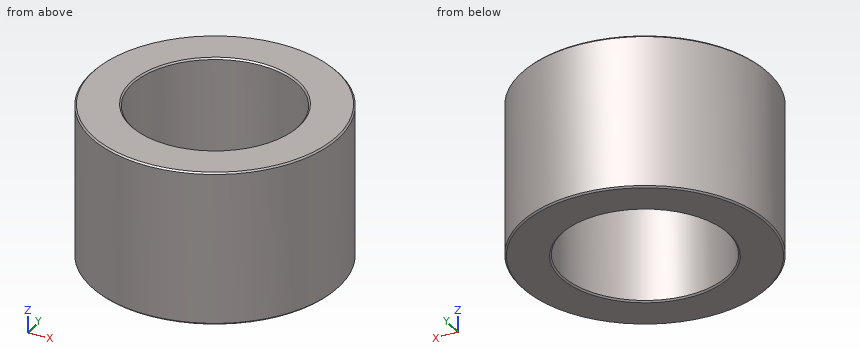
```python
from build123d import *

# Parameters (mm, degrees)
F0_R     = 40.239299
F1_DEPTH = 50
F2_R     = 26.870231
F3_DEPTH = 62
F4_SIZE  = 0.5


with BuildPart() as f1:
    # F0 (on Top) → F1 (new body)
    with BuildSketch(Plane.XY):
        Circle(F0_R)
    extrude(amount=F1_DEPTH)

    # F2 (on face) → F3 (cut)
    with BuildSketch(Plane.XY.offset(50)):
        Circle(F2_R)
    extrude(amount=-F3_DEPTH, mode=Mode.SUBTRACT)

    # F4
    f4_edges = [f1.edges().sort_by_distance(p)[0] for p in [
        (-40.239299, 0, 50),
        (-26.870231, 0, 50),
        (-40.239299, 0, 0),
        (-26.870231, 0, 0),
    ]]
    chamfer(f4_edges, length=F4_SIZE)


solid = f1.part
```
Here's how the part is built. I have some questions about the finished solid (model axes, mm). Round coordinates to 2 decimals unless told otherwise and drop trailing zeros. Write each loop counter-clockwise with the first axis right and the second up, starting at its lowest first coordinate (ties: lowest second). Pieces come first, ordered by that corner, then holes. Notation, with made-up numbers: M 25,77 L 83,77 A23 ccw 83,95 Z; hole C 65.5,62.25 d6. An arc over 180 degrees is marked long. Answer as CSV lines item,"result". Start each with the question number.
1. Suppose I cut it at C-C on z = 7. Write out the boundary of the cut face in (x, y).
2. I'm going to push flat-ended pins straight in: pin 1 Ø2 at (y, z) = (-7.5, 10.5) entering from -X; pin 2 Ø1.5 at (x, z) = (-19, 11) entering from +Y; pin 3 Ø4 at (x, z) = (-16, 20) entering from +Y. Where does each tip first touch, or does it pass through?
3. I need wall thicknesses on probe 1 along Y at (x, z) = (0, 39); probe 2 along Y at (x, z) = (-10, 21.5); probe 3 along X at (y, z) = (-21, 37). Which ranges of each line are inside material? Lowest first, please.
4. Suppose I cut it at A-A on y = 0. Write out the boundary of the cut face in (x, z).
Check result:
1,outline,"C 0,0 d80.48; hole C 0,0 d53.74"
2,pin 1,"stops at x = -39.71"
2,pin 2,"stops at y = 35.86"
2,pin 3,"stops at y = 37.73"
3,probe 1,"y = -40.24 to -26.87, 26.87 to 40.24"
3,probe 2,"y = -38.98 to -24.94, 24.94 to 38.98"
3,probe 3,"x = -34.32 to -16.76, 16.76 to 34.32"
4,outline,"M -40.24,0.5 L -39.74,0 L -27.37,0 L -26.87,0.5 L -26.87,49.5 L -27.37,50 L -39.74,50 L -40.24,49.5 Z; M 26.87,0.5 L 27.37,0 L 39.74,0 L 40.24,0.5 L 40.24,49.5 L 39.74,50 L 27.37,50 L 26.87,49.5 Z"
